Check sheet for the modelled part. Datum: model origin and axes. Units: mm. A direction names the side the tool comes from. Coordinates: 2 decimals unless noted, no trailing zeros. Write each loop counter-clockwise with the first axis right and the second up, starting at its lowest first coordinate (ties: lowest second). Pieces come first, ordered by that corner, then holes. Notation, with made-up numbers: (6.5, 39.5) - (40.5, 39.5) arc R26 ccw to (40.5, 58.5) - close; hole circle Ø7 at (-20, 8.25). An arc over 180 degrees is marked (long way). Use one line per item in the form item = value. Start each with the question number.
1. Tool access check on faces 1 (the face through (31, -5, 80)), 2 (the face through (62, -5, 90)), 3 (the face through (169, -5, 20)). Record the directions out of +Z, -Z, +X, -X, +Y, -Y that give a thin tool (end or side, any length) a straight path to the whole face; none if there is none.
2. Cross-section at A-A on y = -6. Record the boundary of the cut face in (x, z), then the cut area to 3 significant figures.
3. Cross-section at B-B on x = 180. Record the boundary of the cut face in (y, z), then the cut area to 3 significant figures.
4. Cross-section at D-D on z = 32.5. Record the boundary of the cut face in (x, y).
5. Scan lines: line 1 along X through (y, z) = (3.7, 89.79) (3 decimals); line 2 along Y through (x, z) = (52.5, 22); line 3 along X through (y, z) = (-2.75, 94). Record each from-to range of solid material in increasing order.
6. Cross-section at C-C on z = 15.5. Record the boundary of the cut face in (x, y), then the cut area to 3 significant figures.
7. Go/stop test with flat-tipped pins: pin 1 Ø10 at (x, z) = (102, 19) entering from -Y; pin 2 Ø5 at (y, z) = (-4.5, 10) entering from -X; pin 3 Ø1.3 at (x, z) = (133.535, 89.79) entering from -Y; pin 4 Ø3 at (x, y) = (155, -2.5) entering from +Z. Record where each tip stops, or that it passes through.
```python
from build123d import *

# Parameters (mm, degrees)
SKETCH2_W           = 200
SKETCH2_H           = 100
BOSS_EXTRUDE1_DEPTH = 6
SKETCH3_R           = 1.1
CUT_EXTRUDE1_DEPTH  = 6
SKETCH4_W           = 62
SKETCH4_H           = 20
BOSS_EXTRUDE2_DEPTH = 10


with BuildPart() as part:
    # Sketch2 → Boss-Extrude1 (new body)
    with BuildSketch(Plane(origin=(0, 0, 0), x_dir=(1, 0, 0), z_dir=(0, 1, 0))):
        with Locations((100, -50)):
            Rectangle(SKETCH2_W, SKETCH2_H)
    extrude(amount=BOSS_EXTRUDE1_DEPTH)

    # Sketch3 → Cut-Extrude1 (cut)
    with BuildSketch(Plane(origin=(0, 6, 0), x_dir=(1, 0, 0), z_dir=(0, 1, 0))):
        with Locations(Location((66.465, -10.21, 0), (0, 0, 270))):
            Circle(SKETCH3_R)
        with Locations(Location((133.535, -10.21, 0), (0, 0, 270))):
            Circle(SKETCH3_R)
    cut_extrude1 = extrude(amount=-CUT_EXTRUDE1_DEPTH, mode=Mode.SUBTRACT)

    # Mirror1: Cut-Extrude1 across plane
    add(cut_extrude1.mirror(Plane.XY.offset(50)), mode=Mode.SUBTRACT)

    # Sketch4 → Boss-Extrude2 (add)
    with BuildSketch(Plane.XZ):
        with Locations((31, 90)):
            Rectangle(SKETCH4_W, SKETCH4_H)
        with Locations((169, 10)):
            Rectangle(SKETCH4_W, SKETCH4_H)
    extrude(amount=BOSS_EXTRUDE2_DEPTH)


solid = part.part
```
Final values:
q1.face_1 = -Z, +X, -X, -Y
q1.face_2 = +Z, -Z, +X, -Y
q1.face_3 = +Z, +X, -X, -Y
q2.outline = (0, 80) - (62, 80) - (62, 100) - (0, 100) - close; (138, 0) - (200, 0) - (200, 20) - (138, 20) - close
q2.area = 2,480 mm²
q3.outline = (-10, 0) - (6, 0) - (6, 100) - (0, 100) - (0, 20) - (-10, 20) - close
q3.area = 800 mm²
q4.outline = (0, 0) - (200, 0) - (200, 6) - (0, 6) - close
q5.line_1 = 0 to 65.365, 67.565 to 132.435, 134.635 to 200
q5.line_2 = 0 to 6
q5.line_3 = 0 to 62
q6.outline = (0, 0) - (138, 0) - (138, -10) - (200, -10) - (200, 6) - (0, 6) - close
q6.area = 1,820 mm²
q7.pin_1 = 0
q7.pin_2 = 138
q7.pin_3 = through
q7.pin_4 = 20
